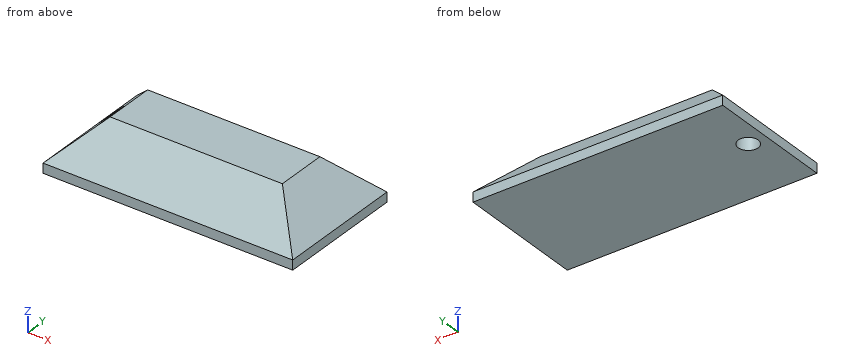
```python
from build123d import *

# Parameters (mm, degrees)
F0_W        = 129.0121003985
F0_H        = 66.4112940431
F1_DEPTH    = 25
F2_R        = 5.1578241127
F3_DEPTH    = 25
F4_T1_DEPTH = 231.8794199172
F4_T3_DEPTH = 169.2786135617


# Not quite as in the source:
# - a fillet or chamfer that OpenCascade refuses, or shapes differently, is made with other operations: its cross-section is extruded or revolved along the edge and cut away or added


with BuildPart() as f1:
    # F0 (on Top) → F1 (new body)
    with BuildSketch(Plane.XY):
        with Locations((1.633066684, 0.4536285996)):
            Rectangle(F0_W, F0_H)
    extrude(amount=F1_DEPTH)

    # F2 (on face) → F3 (cut)
    with BuildSketch(Plane.XY.offset(25)):
        with Locations((-53.4375011921, 2.8125003446)):
            Circle(F2_R)
    extrude(amount=-F3_DEPTH, mode=Mode.SUBTRACT)

    # F4: chamfer of 20 on 4 edges, made by hand

    # F4_s2 → F4_t1 (cut)
    with BuildSketch(Plane.YZ.offset(-114.3066432746)):
        Polygon((-12.7520184219, 25), (-32.7520184219, 5), (-32.7520184219, 25), align=None)
        Polygon((33.6592756212, 5), (13.6592756212, 25), (33.6592756212, 25), align=None)
    extrude(amount=F4_T1_DEPTH, mode=Mode.SUBTRACT)

    # F4_s4 → F4_t3 (cut)
    with BuildSketch(Plane.XZ.offset(-85.0929353805)):
        Polygon((-62.8729835153, 5), (-42.8729835153, 25), (-62.8729835153, 25), align=None)
        Polygon((66.1391168833, 5), (46.1391168833, 25), (66.1391168833, 25), align=None)
    extrude(amount=F4_T3_DEPTH, mode=Mode.SUBTRACT)


solid = f1.part
```
The model under review builds one solid part; all positions refer to its coordinate system, in mm. Coordinates: 2 decimals unless noted, no trailing zeros. Write each loop counter-clockwise with the first axis right and the second up, starting at its lowest first coordinate (ties: lowest second). Pieces come first, ordered by that corner, then holes.
1) We need section C-C on y = 24. State the section outline as (x, z) points.
2) Clearance check with flat-ended pins moving along their axes: pin 1 Ø2 at (x, z) = (-18, 20) entering from -Y; pin 2 Ø6 at (x, y) = (28.5, 24) entering from +Z; pin 3 Ø3 at (y, z) = (13, 10) entering from -X. State where each tip first meets the part, or that it passes through.
3) We need section B-B on z = 8.75. State the section outline as (x, y) points, then the cut area to 3 significant figures.
4) We need section A-A on x = 27. State the section outline as (y, z) points.
5) To check wall thickness, follow probe 1 along Y at (x, z) = (57, 7.25); probe 2 along Z at (x, y) = (-2, -28); probe 3 along Y at (x, z) = (50, 12.75). State the ranges of each line that lie inside material, in increasing order.
6) We need section D-D on z = 22.25. State the section outline as (x, y) points.
Answer list:
1. outline: (-62.87, 0) - (66.14, 0) - (66.14, 5) - (56.48, 14.66) - (-53.21, 14.66) - (-62.87, 5) - close
2. pin 1: stops at y = -18.75
2. pin 2: stops at z = 17.66
2. pin 3: stops at x = -59.37
3. outline: (-59.12, -29) - (62.39, -29) - (62.39, 29.91) - (-59.12, 29.91) - close; hole circle Ø10.32 at (-53.44, 2.81)
3. area: 7,070 mm2
4. outline: (-32.75, 0) - (33.66, 0) - (33.66, 5) - (13.66, 25) - (-12.75, 25) - (-32.75, 5) - close
5. probe 1: y = -30.5 to 31.41
5. probe 2: z = 0 to 9.75
5. probe 3: y = -25 to 25.91
6. outline: (-45.62, -15.5) - (48.89, -15.5) - (48.89, 16.41) - (-45.62, 16.41) - close
